The model under review builds one solid part; all positions refer to its coordinate system, in mm. Face numbers are marked on the shaded views. A direction names the side the tool comes from. Round coordinates to 2 decimals unless told otherwise and drop trailing zeros. Loops run counter-clockwise (first coordinate to the right, second up) from the corner with the lowest first, then second, coordinate; pieces in that order, holes last. Notation, with made-up numbers: M -31,85 L 12,85 A18 ccw 12,97 Z; hole C 63,-6.75 d9. An arc over 180 degrees is marked long. Return JSON: item names as keys, results as strings. Group by question number.
Q1. Consider section D-D (z = -7.5). State the section outline as (x, y) points, and give its area (3 significant figures).
Q2. For the marked faces 5, 6 and 7, list the 3-axis set-ups (+Z, -Z, +X, -X, +Y, -Y) from which the entire face can be reached by the end or side of a thin tool; tool diameter is ignored.
Q3. Consider section A-A (z = 0). State the section outline as (x, y) points, and give its area (3 significant figures).
Q4. Clearance check with flat-ended pins moving along their axes: pin 1 Ø0.9 at (x, y) = (32, 6) entering from -Z; pin 2 Ø23 at (x, z) = (-30, 0) entering from +Y; pin 3 Ø4.5 at (x, y) = (-30.5, 7) entering from +Z; pin 4 Ø5 at (y, z) = (14.5, 1) entering from +X. State where each tip first meets the part, or that it passes through.
Q5. Consider section B-B (x = -30). State the section outline as (y, z) points.
Q6. Consider section C-C (z = -17.5). State the section outline as (x, y) points.
Q7. To check wall thickness, follow line 1 along Z through (x, y) = (-14, 13.5); line 2 along X through (y, z) = (11.5, 12.5); line 3 along Z through (x, y) = (26.15, 7.5). State the ranges of each line that lie inside material, in increasing order.
Q8. Draft analysis for pull direction Z (two halves, no side actions). For the marked faces 1, 2, 3 and 4, state which applies: pulls with the +Z half, pulls with the -Z half, needs draft (parallel to the pull), parting line crosses it, or undercut.
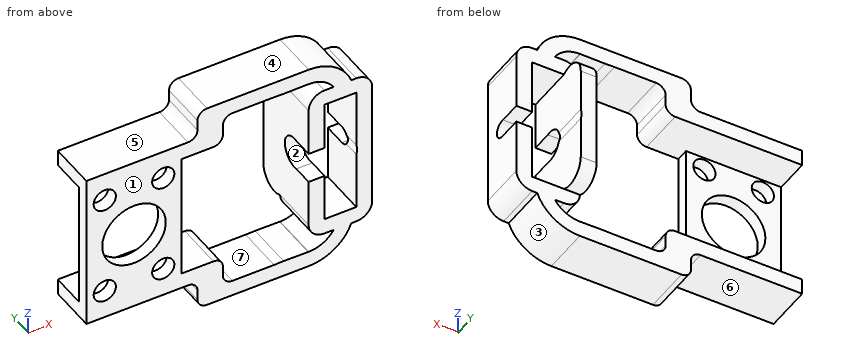
from build123d import *

# Parameters (mm, degrees)
SKETCH1_W           = 90
SKETCH1_H           = 50
BOSS_EXTRUDE1_DEPTH = 15
SKETCH2_W           = 40
SKETCH2_H           = 40
SKETCH2_W_2         = 10
CUT_EXTRUDE1_DEPTH  = 15
SKETCH6_R           = 2.75
CUT_EXTRUDE4_DEPTH  = 7
SKETCH8_R           = 5
CUT_EXTRUDE5_DEPTH  = 7
BOSS_EXTRUDE2_DEPTH = 15
SKETCH11_W          = 7.860960604
SKETCH11_H          = 5
CUT_EXTRUDE7_DEPTH  = 15
FILLET1_R           = 5
FILLET2_R           = 5
FILLET3_R           = 5
FILLET4_R           = 5
FILLET5_R           = 5
SKETCH12_W          = 6.801796193
SKETCH12_H          = 5.5
CUT_EXTRUDE8_DEPTH  = 7.5
SKETCH13_W          = 7.647159446
SKETCH13_H          = 9.789246186
CUT_EXTRUDE9_DEPTH  = 7.5
BOSS_EXTRUDE4_DEPTH = 5
SKETCH16_W          = 30
SKETCH16_H          = 40
CUT_EXTRUDE10_DEPTH = 5
SKETCH18_R          = 10
SKETCH18_R_2        = 3.5
CUT_EXTRUDE12_DEPTH = 11
SKETCH17_R          = 5.25
CUT_EXTRUDE13_DEPTH = 32
BOSS_EXTRUDE5_DEPTH = 15
CUT_EXTRUDE14_DEPTH = 15
FILLET7_R           = 3
SKETCH21_W          = 40
SKETCH21_H          = 6
CUT_EXTRUDE15_DEPTH = 30


with BuildPart() as part:
    # Sketch1 → Boss-Extrude1 (new body)
    with BuildSketch(Plane(origin=(0, 0, 0), x_dir=(1, 0, 0), z_dir=(0, 1, 0))):
        Rectangle(SKETCH1_W, SKETCH1_H)
    extrude(amount=BOSS_EXTRUDE1_DEPTH)

    # Sketch2 → Cut-Extrude1 (cut)
    with BuildSketch(Plane(origin=(0, 15, 0), x_dir=(1, 0, 0), z_dir=(0, 1, 0))):
        with Locations((5, 0)):
            Rectangle(SKETCH2_W, SKETCH2_H)
        with Locations((35, 0)):
            Rectangle(SKETCH2_W_2, SKETCH2_H)
    extrude(amount=-CUT_EXTRUDE1_DEPTH, mode=Mode.SUBTRACT)

    # Sketch6 → Cut-Extrude4 (cut)
    with BuildSketch(Plane(origin=(45, 0, 0), x_dir=(0, 0, -1), z_dir=(1, 0, 0))):
        with Locations((0, 7.5)):
            Circle(SKETCH6_R)
    extrude(amount=-CUT_EXTRUDE4_DEPTH, mode=Mode.SUBTRACT)

    # Sketch8 → Cut-Extrude5 (cut)
    with BuildSketch(Plane.ZY.offset(-25)):
        with Locations((0, 7.5)):
            Circle(SKETCH8_R)
    extrude(amount=-CUT_EXTRUDE5_DEPTH, mode=Mode.SUBTRACT)

    # Sketch10 → Boss-Extrude2 (add)
    with BuildSketch(Plane(origin=(0, 15, 0), x_dir=(1, 0, 0), z_dir=(0, 1, 0))):
        with BuildLine():
            Line((11.563534407, 25), (17.139039396, 25))
            ThreePointArc((17.139039396, 25), (20.515980342, 28.166288589), (25, 29.316367404))
            ThreePointArc((25, 29.316367404), (29.484019658, 28.166288589), (32.860960604, 25))
            Line((32.860960604, 25), (38.436465593, 25))
            ThreePointArc((38.436465593, 25), (33.180938792, 31.773310839), (25, 34.336617719))
            ThreePointArc((25, 34.336617719), (16.819061208, 31.773310839), (11.563534407, 25))
        make_face()
        with BuildLine():
            Line((11.563534407, -25), (17.139039396, -25))
            ThreePointArc((17.139039396, -25), (20.515980342, -28.166288589), (25, -29.316367404))
            ThreePointArc((25, -29.316367404), (29.484019658, -28.166288589), (32.860960604, -25))
            Line((32.860960604, -25), (38.436465593, -25))
            ThreePointArc((38.436465593, -25), (33.180938792, -31.773310839), (25, -34.336617719))
            ThreePointArc((25, -34.336617719), (16.819061208, -31.773310839), (11.563534407, -25))
        make_face()
    extrude(amount=-BOSS_EXTRUDE2_DEPTH)

    # Sketch11 → Cut-Extrude7 (cut)
    with BuildSketch(Plane(origin=(0, 15, 0), x_dir=(1, 0, 0), z_dir=(0, 1, 0))):
        with Locations((21.069519698, 22.5)):
            Rectangle(SKETCH11_W, SKETCH11_H)
        with Locations((21.069519698, -22.5)):
            Rectangle(SKETCH11_W, SKETCH11_H)
    extrude(amount=-CUT_EXTRUDE7_DEPTH, mode=Mode.SUBTRACT)

    # Fillet1
    fillet1_edges = [part.edges().sort_by_distance(p)[0] for p in [
        (25, 7.5, 25),
        (25, 7.5, -25),
    ]]
    fillet(fillet1_edges, radius=FILLET1_R)

    # Fillet2
    fillet2_edges = [part.edges().sort_by_distance(p)[0] for p in [
        (17.139039396, 7.5, 20),
        (17.139039396, 7.5, -20),
    ]]
    fillet(fillet2_edges, radius=FILLET2_R - 0.0001)  # a hair under: the kernel refuses the full size

    # Fillet3
    fillet3_edges = [part.edges().sort_by_distance(p)[0] for p in [
        (17.139039396, 7.5, -25),
        (17.139039396, 7.5, 25),
    ]]
    fillet(fillet3_edges, radius=FILLET3_R)

    # Fillet4
    fillet4_edges = [part.edges().sort_by_distance(p)[0] for p in [
        (45, 7.5, 25),
        (45, 7.5, -25),
    ]]
    fillet(fillet4_edges, radius=FILLET4_R)

    # Fillet5
    fillet5_edges = [part.edges().sort_by_distance(p)[0] for p in [
        (11.563534407, 7.5, -25),
        (11.563534407, 7.5, 25),
    ]]
    fillet(fillet5_edges, radius=FILLET5_R)

    # Sketch12 → Cut-Extrude8 (cut)
    with BuildSketch(Plane(origin=(0, 15, 0), x_dir=(1, 0, 0), z_dir=(0, 1, 0))):
        with Locations((42.246807925, 0.040811044)):
            Rectangle(SKETCH12_W, SKETCH12_H)
    extrude(amount=-CUT_EXTRUDE8_DEPTH, mode=Mode.SUBTRACT)

    # Sketch13 → Cut-Extrude9 (cut)
    with BuildSketch(Plane.XZ):
        with Locations((27.507381734, 0)):
            Rectangle(SKETCH13_W, SKETCH13_H)
    extrude(amount=-CUT_EXTRUDE9_DEPTH, mode=Mode.SUBTRACT)

    # Sketch15 → Boss-Extrude4 (add)
    with BuildSketch(Plane(origin=(30, 0, 0), x_dir=(0, 0, -1), z_dir=(1, 0, 0))):
        with BuildLine():
            Line((-15, 23.80846108), (15, 23.80846108))
            ThreePointArc((15, 23.80846108), (20.064311074, 20.859825933), (20, 15))
            Line((20, 15), (-20, 15))
            ThreePointArc((-20, 15), (-20.064311074, 20.859825933), (-15, 23.80846108))
        make_face()
    extrude(amount=-BOSS_EXTRUDE4_DEPTH)

    # Sketch16 → Cut-Extrude10 (cut)
    with BuildSketch(Plane(origin=(0, 15, 0), x_dir=(1, 0, 0), z_dir=(0, 1, 0))):
        with Locations((-30, 0)):
            Rectangle(SKETCH16_W, SKETCH16_H)
    extrude(amount=-CUT_EXTRUDE10_DEPTH, mode=Mode.SUBTRACT)

    # Sketch18 → Cut-Extrude12 (cut)
    with BuildSketch(Plane(origin=(0, 10, 0), x_dir=(1, 0, 0), z_dir=(0, 1, 0))):
        with Locations(Location((-30, 0, 0), (0, 0, 270))):
            Circle(SKETCH18_R)
        with Locations(Location((-39.206960866, 15.841368379, 0), (0, 0, 270))):
            Circle(SKETCH18_R_2)
        with Locations(Location((-20.793039134, 15.841368379, 0), (0, 0, 270))):
            Circle(SKETCH18_R_2)
        with Locations(Location((-20.793039134, -15.841368379, 0), (0, 0, 270))):
            Circle(SKETCH18_R_2)
        with Locations(Location((-39.206960866, -15.841368379, 0), (0, 0, 270))):
            Circle(SKETCH18_R_2)
    extrude(amount=-CUT_EXTRUDE12_DEPTH, mode=Mode.SUBTRACT)

    # Sketch17 → Cut-Extrude13 (cut)
    with BuildSketch(Plane(origin=(0, 23.80846108, 0), x_dir=(1, 0, 0), z_dir=(0, 1, 0))):
        with Locations((35, 0)):
            Circle(SKETCH17_R)
    extrude(amount=-CUT_EXTRUDE13_DEPTH, mode=Mode.SUBTRACT)

    # Sketch19 → Boss-Extrude5 (add)
    with BuildSketch(Plane(origin=(0, 15, 0), x_dir=(1, 0, 0), z_dir=(0, 1, 0))):
        Polygon((25, 34.336617719), (-10, 34.336617719), (-10, 25), (-2, 25), (-2, 29.316367404), (25, 29.316367404), align=None)
        Polygon((-2, -29.316367404), (-2, -25), (-10, -25), (-10, -34.336617719), (25, -34.336617719), (25, -29.316367404), align=None)
    extrude(amount=-BOSS_EXTRUDE5_DEPTH)

    # Sketch20 → Cut-Extrude14 (cut)
    with BuildSketch(Plane(origin=(0, 15, 0), x_dir=(1, 0, 0), z_dir=(0, 1, 0))):
        Polygon((-2, -25), (-2, -20), (17.115013572, -20), (25, -29.316367404), (17.115013572, -29.241305009), (14.103032256, -29.316367404), align=None)
        Polygon((17.115013572, 29.241305009), (14.103032256, 29.316367404), (-2, 25), (-2, 20), (17.115013572, 20), (25, 29.316367404), align=None)
    extrude(amount=-CUT_EXTRUDE14_DEPTH, mode=Mode.SUBTRACT)

    # Fillet7
    fillet7_edges = [part.edges().sort_by_distance(p)[0] for p in [
        (-2, 7.5, -29.316367404),
        (-10, 7.5, -25),
        (-10, 7.5, -34.336617719),
        (-2, 7.5, 29.316367404),
        (-10, 7.5, 34.336617719),
        (-10, 7.5, 25),
        (-2, 7.5, 20),
        (-2, 7.5, -20),
    ]]
    fillet(fillet7_edges, radius=FILLET7_R)

    # Sketch21 → Cut-Extrude15 (cut)
    with BuildSketch(Plane.ZY.offset(45)):
        with Locations((0, 7)):
            Rectangle(SKETCH21_W, SKETCH21_H)
    extrude(amount=-CUT_EXTRUDE15_DEPTH, mode=Mode.SUBTRACT)


solid = part.part
Values:
{
 "1": {"outline": "M -45,0 L -36.61,0 L -36.61,4 L -45,4 Z; M -23.39,0 L -15,0 L -15,4 L -23.39,4 Z; M 25,0 L 30,0 L 30,23.81 L 25,23.81 Z; M 40,0 L 45,0 L 45,15 L 40,15 Z", "area": "261 mm2"},
 "2": {"face 5": "+Z, -X, +Y, -Y", "face 6": "-Z, -X, +Y, -Y", "face 7": "+Y, -Y"},
 "3": {"outline": "M -45,0 L -40,0 L -40,4 L -45,4 Z; M -20,0 L -15,0 L -15,4 L -20,4 Z; M 25,12.5 L 29.75,12.5 L 29.75,23.81 L 25,23.81 Z; M 40.25,0 L 45,0 L 45,4.75 L 40.25,4.75 Z", "area": "116 mm2"},
 "4": {"pin 1": "stops at z = -32.75", "pin 2": "stops at y = 4", "pin 3": "stops at z = 25", "pin 4": "stops at x = 45"},
 "5": {"outline": "M 0,-25 L 15,-25 L 15,-20 L 4,-20 L 4,-10 L 0,-10 Z; M 0,10 L 4,10 L 4,20 L 15,20 L 15,25 L 0,25 Z"},
 "6": {"outline": "M -45,0 L -42.29,0 L -42.29,4 L -45,4 Z; M -36.12,0 L -23.88,0 L -23.88,4 L -36.12,4 Z; M -17.71,0 L -15,0 L -15,4 L -17.71,4 Z; M 25,0 L 30,0 L 30,23.24 L 25,23.24 Z; M 40,0 L 45,0 L 45,15 L 40,15 Z"},
 "7": {"line 1": "z = -25 to -20, 20 to 25", "line 2": "x = 25 to 30, 40 to 45", "line 3": "z = -34.29 to -29.25, -23.19 to -5, 5 to 23.19, 29.25 to 34.29"},
 "8": {"face 1": "needs draft", "face 2": "undercut", "face 3": "pulls with the -Z half", "face 4": "pulls with the +Z half"}
}
